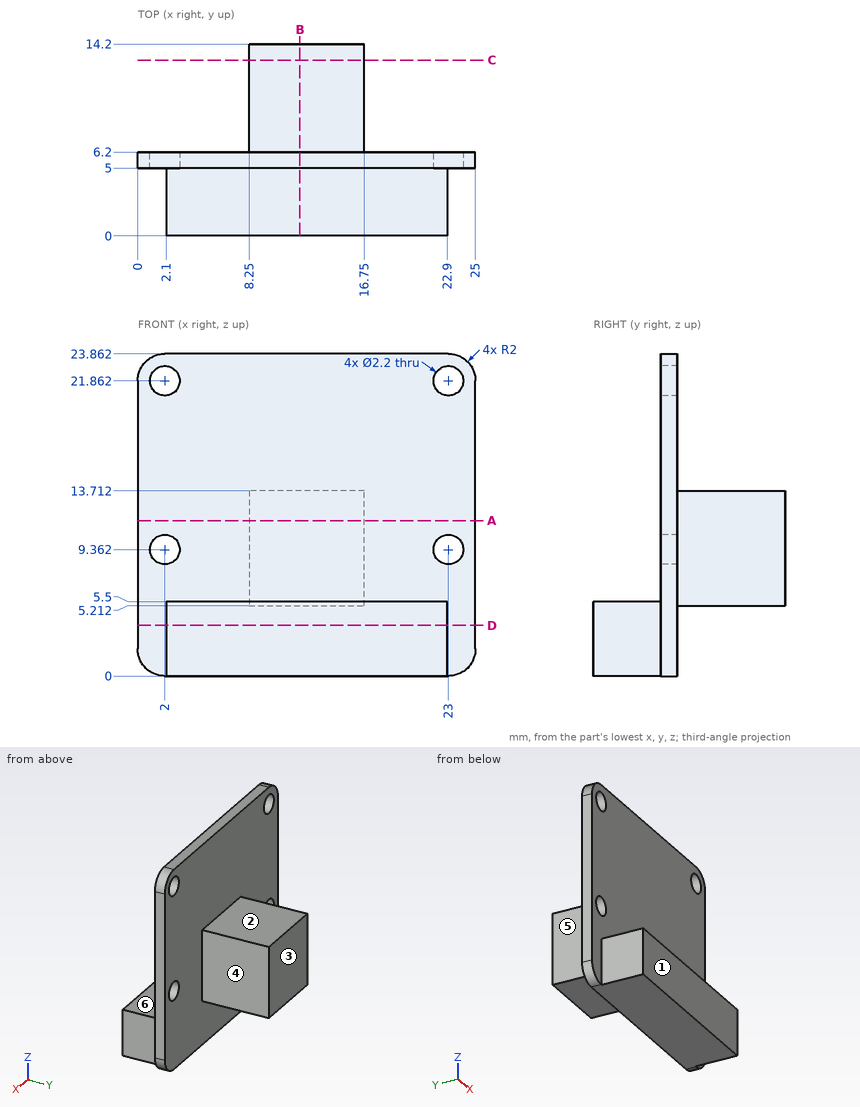
Design review of the part shown in the three views and the two pictorial views. Dimensions are in mm from the part's minimum x, y and z. A direction names the side the tool comes from. Round coordinates to 2 decimals unless told otherwise and drop trailing zeros. Order: outer loops, then holes, each group sorted by start corner. A loop starts at its lowest first (then second) coordinate and runs counter-clockwise, first axis right, second up.
(1) Tool access review of the marked faces 4, 5 and 6: name each direction out of +Z, -Z, +X, -X, +Y, -Y from which nothing blocks a thin tool from reaching the whole face with its end or side.
Working result:
face 4: +Z, -Z, +X, +Y
face 5: +Z, -Z, -X, +Y
face 6: +Z, +X, -X, -Y
(2) Wall thickness on L1, parallel to Z at x = 23, y = 5.8; L2, parallel to Y at x = 6.25, z = 15; L3, parallel to X at y = 1, z = 3.5: over which ranges is each line inside the solid? List them lowest first.
Working result:
L1: z = 0 to 8.26, 10.46 to 20.76, 22.96 to 23.86
L2: y = 5 to 6.2
L3: x = 2.1 to 22.9
(3) Take a section at B-B, the plane x = 12. State the section outline as (y, z) points, plus the area to 3 significant figures.
Working result:
outline: (0, 0) - (6.2, 0) - (6.2, 5.21) - (14.2, 5.21) - (14.2, 13.71) - (6.2, 13.71) - (6.2, 23.86) - (5, 23.86) - (5, 5.5) - (0, 5.5) - close
area: 124 mm2
(4) Take a section at D-D, the plane z = 3.75. State the section outline as (x, y) points.
Working result:
outline: (0, 5) - (2.1, 5) - (2.1, 0) - (22.9, 0) - (22.9, 5) - (25, 5) - (25, 6.2) - (0, 6.2) - close
(5) For P1, Ø10, axis at x = 18, z = 3.5, coming from the -Y side; P2, Ø6.5, axis at y = 10.5, z = 7.5, coming from the -X side; P3, Ø2.5, axis at x = 2, z = 21.862, coming from the -Y side; P4, Ø2, axis at y = 3.5, z = 5, coming from the +X side, all flat-tipped, find the tip position at first contact; note any pin that passes through.
Working result:
P1: stops at y = 0
P2: stops at x = 8.25
P3: stops at y = 5
P4: stops at x = 22.9
(6) Take a section at A-A, the plane z = 11.5. State the section outline as (x, y) points, plus the area to 3 significant figures.
Working result:
outline: (0, 5) - (25, 5) - (25, 6.2) - (16.75, 6.2) - (16.75, 14.2) - (8.25, 14.2) - (8.25, 6.2) - (0, 6.2) - close
area: 98.0 mm2
(7) Take a section at C-C, the plane y = 13. State the section outline as (x, z) points, plus the area to 4 significant figures.
Working result:
outline: (8.25, 5.21) - (16.75, 5.21) - (16.75, 13.71) - (8.25, 13.71) - close
area: 72.25 mm2
(8) Mouldability with a two-part tool opening along Y and no side actions: class the marked faces 1, 2 and 3 as released by +Y, released by -Y, zero draft, split by the parting line, or undercut.
Working result:
face 1: released by -Y
face 2: zero draft
face 3: released by +Y
